```python
from build123d import *

# Parameters (mm, degrees)
F1_DEPTH = 60
F2_W     = 48
F2_H     = 28.6153249443
F3_DEPTH = 170.001
F4_W     = 55
F4_H     = 48
F5_DEPTH = 5
F7_DEPTH = 30.001


with BuildPart() as f1:
    # F0 (on Front) → F1 (new body)
    with BuildSketch(Plane.XZ):
        with BuildLine():
            Line((-70, -7.5), (-70, -12.5))
            Line((-70, -12.5), (-35, -12.5))
            Line((-35, -12.5), (-35, -2.5))
            ThreePointArc((-35, -2.5), (-33.5355339059, 1.0355339059), (-30, 2.5))
            Line((-30, 2.5), (30, 2.5))
            ThreePointArc((30, 2.5), (33.5355339059, 1.0355339059), (35, -2.5))
            Line((35, -2.5), (35, -12.5))
            Line((35, -12.5), (70, -12.5))
            Line((70, -12.5), (70, -7.5))
            ThreePointArc((70, -7.5), (71.4644660941, -3.9644660941), (75, -2.5))
            Line((75, -2.5), (85, -2.5))
            Line((85, -2.5), (85, 12.5))
            Line((85, 12.5), (-85, 12.5))
            Line((-85, 12.5), (-85, -2.5))
            Line((-85, -2.5), (-75, -2.5))
            ThreePointArc((-75, -2.5), (-71.4644660941, -3.9644660941), (-70, -7.5))
        make_face()
        with BuildLine():
            ThreePointArc((85, 12.5), (0, 38.9079290569), (-85, 12.5))
            Line((-85, 12.5), (85, 12.5))
        make_face()
    extrude(amount=F1_DEPTH)

    # F2 (on face) → F3 (cut, through all)
    with BuildSketch(Plane.YZ.offset(85)):
        with Locations((-30, 26.8076624721)):
            Rectangle(F2_W, F2_H)
    extrude(amount=-F3_DEPTH, mode=Mode.SUBTRACT)

    # F4 (on face) → F5 (join)
    with BuildSketch(Plane.XY.offset(12.5)):
        with Locations((0, -30)):
            Rectangle(F4_W, F4_H)
    extrude(amount=F5_DEPTH)

    # F6 (on face) → F7 (cut, through all)
    with BuildSketch(Plane.XY.offset(17.5)):
        with BuildLine():
            ThreePointArc((0, -30), (-2.9289321881, -37.0710678119), (-10, -40))
            Line((-10, -40), (10, -40))
            ThreePointArc((10, -40), (2.9289321881, -37.0710678119), (0, -30))
        make_face()
        with BuildLine():
            ThreePointArc((-10, -20), (-20, -30), (-10, -40))
            Line((-10, -40), (-10, -20))
        make_face()
        with BuildLine():
            Line((-10, -20), (-10, -40))
            ThreePointArc((-10, -40), (-2.9289321881, -37.0710678119), (0, -30))
            ThreePointArc((0, -30), (-2.9289321881, -22.9289321881), (-10, -20))
        make_face()
        with BuildLine():
            ThreePointArc((0, -30), (2.9289321881, -37.0710678119), (10, -40))
            Line((10, -40), (10, -20))
            ThreePointArc((10, -20), (2.9289321881, -22.9289321881), (0, -30))
        make_face()
        with BuildLine():
            Line((10, -20), (10, -40))
            ThreePointArc((10, -40), (17.0710678119, -37.0710678119), (20, -30))
            ThreePointArc((20, -30), (17.0710678119, -22.9289321881), (10, -20))
        make_face()
        with BuildLine():
            Line((10, -20), (-10, -20))
            ThreePointArc((-10, -20), (-2.9289321881, -22.9289321881), (0, -30))
            ThreePointArc((0, -30), (2.9289321881, -22.9289321881), (10, -20))
        make_face()
    extrude(amount=-F7_DEPTH, mode=Mode.SUBTRACT)


solid = f1.part
```
Source: CAD feature listing. Evaluate the final solid. Frame: model axes, mm. A direction names the side the tool comes from. Give positions to 0.01 mm unless a question says otherwise; leave off trailing zeros. Write each loop counter-clockwise with the first axis right and the second up, starting at its lowest first coordinate (ties: lowest second). Pieces come first, ordered by that corner, then holes. Notation, with made-up numbers: (67, 80) - (91, 80) arc R24 ccw to (91, 92) - close; hole circle Ø9 at (3, 42). An arc over 180 degrees is marked (long way). One line per item, written item: value. Start each with the question number.
Q1. Section query A-A, the plane z = -4.5. Return the cut outline in (x, y), then the cut area to 3 significant figures.
Q2. Draft query along X for faces 4 (the face through (1, -54, 26)), 5 (the face through (-33.57, -29.58, 1)), 6 (the face through (85, -30, 5)). Return one class per face: +X half, -X half, draft (parallel to the pull), parting line (faces both ways), or undercut.
Q3. Section query B-B, the plane y = -47. Return the cut outline in (x, z).
Q4. First-contact query: pin 1 Ø1.5 at (y, z) = (-31, 14) entering from +X; pin 2 Ø4 at (y, z) = (-44.5, -11) entering from +X; pin 3 Ø1.5 at (y, z) = (-44.5, -9) entering from -X. Flat tips, straight axial feed; report the tip coordinate or a pass-through.
Q5. Section query D-D, the plane x = 52. Return the cut outline in (y, z), then the cut area to 3 significant figures.
Q6. Material intervals for probe 1 along X at (y, z) = (-38, -8.5); probe 2 along Y at (x, z) = (-37, 18.5); probe 3 along Y at (x, z) = (-4, 16), sorted ascending. Write a range as from..to.
Q7. Section query C-C, the plane z = 8. Return the cut outline in (x, y).
Q8. Set-up query: faces 1 (the face through (70, -30, -10)), 2 (the face through (-27.5, -30, 15)), 3 (the face through (27.5, -30, 15)). Return all of +Z, -Z, +X, -X, +Y, -Y with unobstructed straight access to the full face (end or side cutting, diameter ignored); none if empty.
Answer:
1. outline: (-71, -60) - (-35, -60) - (-35, 0) - (-71, 0) - close; (35, -60) - (71, -60) - (71, 0) - (35, 0) - close
1. area: 4,320 mm2
2. face 4: draft
2. face 5: undercut
2. face 6: +X half
3. outline: (-85, -2.5) - (-75, -2.5) arc R5 cw to (-70, -7.5) - (-70, -12.5) - (-35, -12.5) - (-35, -2.5) arc R5 cw to (-30, 2.5) - (30, 2.5) arc R5 cw to (35, -2.5) - (35, -12.5) - (70, -12.5) - (70, -7.5) arc R5 cw to (75, -2.5) - (85, -2.5) - (85, 12.5) - (27.5, 12.5) - (27.5, 17.5) - (-27.5, 17.5) - (-27.5, 12.5) - (-85, 12.5) - close
4. pin 1: stops at x = 27.5
4. pin 2: stops at x = 70
4. pin 3: stops at x = -70
5. outline: (-60, -12.5) - (0, -12.5) - (0, 29.61) - (-6, 29.61) - (-6, 12.5) - (-54, 12.5) - (-54, 29.61) - (-60, 29.61) - close
5. area: 1,710 mm2
6. probe 1: x = -70..-35, 35..70
6. probe 2: y = -60..-54, -6..0
6. probe 3: y = -60..-40, -20..0
7. outline: (-85, -60) - (85, -60) - (85, 0) - (-85, 0) - close; hole (-10, -40) - (10, -40) arc R10 ccw to (10, -20) - (-10, -20) arc R10 ccw to start
8. face 1: -Z, +X, +Y, -Y
8. face 2: +Z, -X
8. face 3: +Z, +X
